Geometry check sheet. Reference: drawing and pictorial views, mm from the part's lowest x, y, z. A direction names the side the tool comes from. Coordinates: 2 decimals unless noted, no trailing zeros. Write each loop counter-clockwise with the first axis right and the second up, starting at its lowest first coordinate (ties: lowest second). Pieces come first, ordered by that corner, then holes. Notation, with made-up numbers: (-23.75, 47) -> (-13.75, 47) arc R17 cw to (-13.75, 78) -> close; hole circle Ø7 at (72, 31.25). An arc over 180 degrees is marked (long way). Answer in a Markdown table with one row per item.
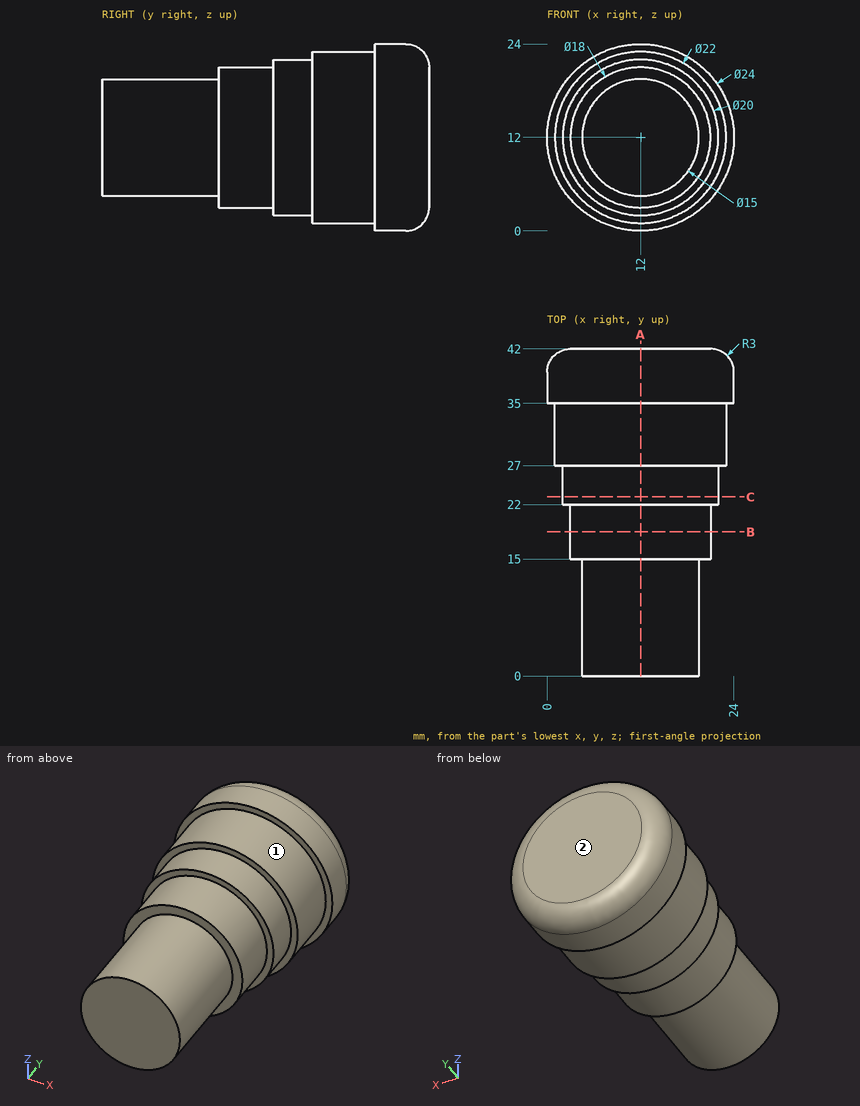
1. Tool access check on the marked faces 1 and 2. Record the directions out of +Z, -Z, +X, -X, +Y, -Y that give a thin tool (end or side, any length) a straight path to the whole face; none if there is none.
Geometry says:
| item | result |
|---|---|
| face 1 | -Y |
| face 2 | +Z, -Z, +X, -X, +Y |
2. Section check C-C, the plane y = 23. Record the boundary of the cut face in (x, z).
Geometry says:
| item | result |
|---|---|
| outline | circle Ø20 at (12, 12) |
3. Thickness scan on line 1 (Y direction, x = 5, z = 7.5); line 2 (Y direction, x = 15.25, z = 22); line 3 (Z direction, x = 20.25, y = 36). Record the ranges inside material, lowest first. Write a range as from..to.
Geometry says:
| item | result |
|---|---|
| line 1 | 15..42 |
| line 2 | 27..41.59 |
| line 3 | 3.29..20.71 |
4. Depth check by flat-ended pin: P1, Ø2, axis at x = 13, z = 2.5, coming from the -Y side; P2, Ø3, axis at y = 15, z = 12.5, coming from the -X side; P3, Ø3, axis at y = 27.5, z = 13.5, coming from the +X side. Enter the tip coordinate at first touch or a pass-through.
Geometry says:
| item | result |
|---|---|
| P1 | y = 15 |
| P2 | x = 3 |
| P3 | x = 23 |
5. Section check A-A, the plane x = 12. Record the boundary of the cut face in (y, z).
Geometry says:
| item | result |
|---|---|
| outline | (0, 4.5) -> (15, 4.5) -> (15, 3) -> (22, 3) -> (22, 2) -> (27, 2) -> (27, 1) -> (35, 1) -> (35, 0) -> (39, 0) arc R3 ccw to (42, 3) -> (42, 21) arc R3 ccw to (39, 24) -> (35, 24) -> (35, 23) -> (27, 23) -> (27, 22) -> (22, 22) -> (22, 21) -> (15, 21) -> (15, 19.5) -> (0, 19.5) -> close |
6. Section check B-B, the plane y = 18.5. Record the boundary of the cut face in (x, z).
Geometry says:
| item | result |
|---|---|
| outline | circle Ø18 at (12, 12) |
